Geometry: final body of the model. Coordinates: model frame, mm. Coordinates: 2 decimals unless noted, no trailing zeros. Write each loop counter-clockwise with the first axis right and the second up, starting at its lowest first coordinate (ties: lowest second). Pieces come first, ordered by that corner, then holes. Notation, with made-up numbers: (88.25, -23.75) - (109.25, -23.75) arc R7 cw to (109.25, -10.75) - close; hole circle Ø7 at (44, 28.25). An arc over 180 degrees is marked (long way). Put each result on its own line as item: value.
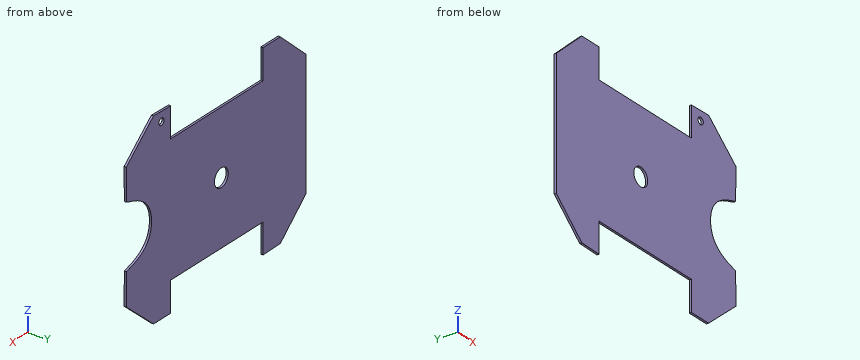
```python
from build123d import *

# Parameters (mm, degrees)
EXTRUDE_1_DEPTH     = 5
SKETCH_2_R          = 21
CUT_EXTRUDE_1_DEPTH = 403.120979525
SKETCH1_R           = 8
CUT_EXTRUDE1_DEPTH  = 403.120979525


with BuildPart() as part:
    # Эскиз1 → Вытянуть1 (new body)
    with BuildSketch(Plane(origin=(0, 0, 0), x_dir=(1, 0, 0), z_dir=(0, 1, 0))):
        with BuildLine():
            Line((-269.7921816, 73.262575573), (-269.7921816, -223.012011978))
            Line((-269.7921816, -223.012011978), (-192.586469874, -293.492830448))
            Line((-192.586469874, -293.492830448), (-140.586469874, -293.492830448))
            Line((-140.586469874, -293.492830448), (-140.586469874, -223.492830448))
            Line((-140.586469874, -223.492830448), (139.068300868, -223.492830448))
            Line((139.068300868, -223.492830448), (139.068300868, -293.492830448))
            Line((139.068300868, -293.492830448), (191.068300868, -294.890935713))
            Line((191.068300868, -294.890935713), (273.341577689, -223.012011978))
            Line((273.341577689, -223.012011978), (273.101729514, -148.382005757))
            add(Edge.make_bspline(
                [(273.101729514, -148.382005757), (239.363891717, -139.145872689), (197.437007815, -125.423723423), (197.047353036, -74.874718203)],
                knots=[0, 0, 0, 0, 1, 1, 1, 1], degree=3))
            add(Edge.make_bspline(
                [(273.101729514, -1.367430648), (239.363891717, -10.603563716), (197.437007815, -24.325712982), (197.047353036, -74.874718203)],
                knots=[0, 0, 0, 0, 1, 1, 1, 1], degree=3))
            Line((273.101729514, -1.367430648), (273.341577689, 73.262575573))
            Line((273.341577689, 73.262575573), (191.068300868, 145.141499308))
            Line((191.068300868, 145.141499308), (139.068300868, 145.141499308))
            Line((139.068300868, 145.141499308), (139.068300868, 75.141499308))
            Line((139.068300868, 75.141499308), (-140.586469874, 75.141499308))
            Line((-140.586469874, 75.141499308), (-140.586469874, 145.141499308))
            Line((-140.586469874, 145.141499308), (-192.586469874, 143.743394043))
            Line((-192.586469874, 143.743394043), (-269.7921816, 73.262575573))
        make_face()
    extrude(amount=EXTRUDE_1_DEPTH)

    # Эскиз2 → Вырез-Вытянуть1 (cut, through all)
    with BuildSketch(Plane(origin=(0, 5, 0), x_dir=(-1, 0, 0), z_dir=(0, 1, 0))):
        with Locations(Location((14.229950912, 74.026657254, 0), (0, 0, 90))):
            Circle(SKETCH_2_R)
    extrude(amount=-CUT_EXTRUDE_1_DEPTH, mode=Mode.SUBTRACT)

    # Sketch1 → Cut-Extrude1 (cut, through all)
    with BuildSketch(Plane(origin=(0, 5, 0), x_dir=(1, 0, 0), z_dir=(0, 1, 0))):
        with Locations(Location((167.052967516, -272.065876514, 0), (0, 0, 270))):
            Circle(SKETCH1_R)
    extrude(amount=-CUT_EXTRUDE1_DEPTH, mode=Mode.SUBTRACT)


solid = part.part
```
1. Ray query, probe 1 along Z at (x, y) = (103, 3); probe 2 along X at (y, z) = (4.1, 212.5); probe 3 along Z at (x, y) = (219, 1.5). Return the intervals inside material, ascending. Write a range as from..to.
Answer below:
probe 1: z = -75.14..223.49
probe 2: x = -269.79..273.31
probe 3: z = -120.74..25.44, 124.31..270.49
2. Section query A-A (z = -114.5). Return loops of the section in (x, y), then the cut area to 3 significant figures.
Answer below:
outline: (-224.62, 0) - (-140.59, 0) - (-140.59, 5) - (-224.62, 5) - close; (139.07, 0) - (226.14, 0) - (226.14, 5) - (139.07, 5) - close
area: 856 mm²
3. Section query B-B (x = 59.5). Return loops of the section in (y, z), then the cut area to 3 significant figures.
Answer below:
outline: (0, -75.14) - (5, -75.14) - (5, 223.49) - (0, 223.49) - close
area: 1,490 mm²
4. Pin query (flat end, axial travel): pin 1 Ø2.5 at (x, y) = (53, 3.5) entering from -Z; pin 2 Ø3 at (x, y) = (-116, 0.5) entering from +Z. Return the tip coordinate at first contact, or that it passes through.
Answer below:
pin 1: stops at z = -75.14
pin 2: stops at z = 223.49
5. Section query C-C (y = 0.95). Count the separate pieces of the cut face and the enclosed holes in it, then the cut area to 3 significant figures.
Answer below:
separate pieces: 1
enclosed holes: 2
area: 178,000 mm²
